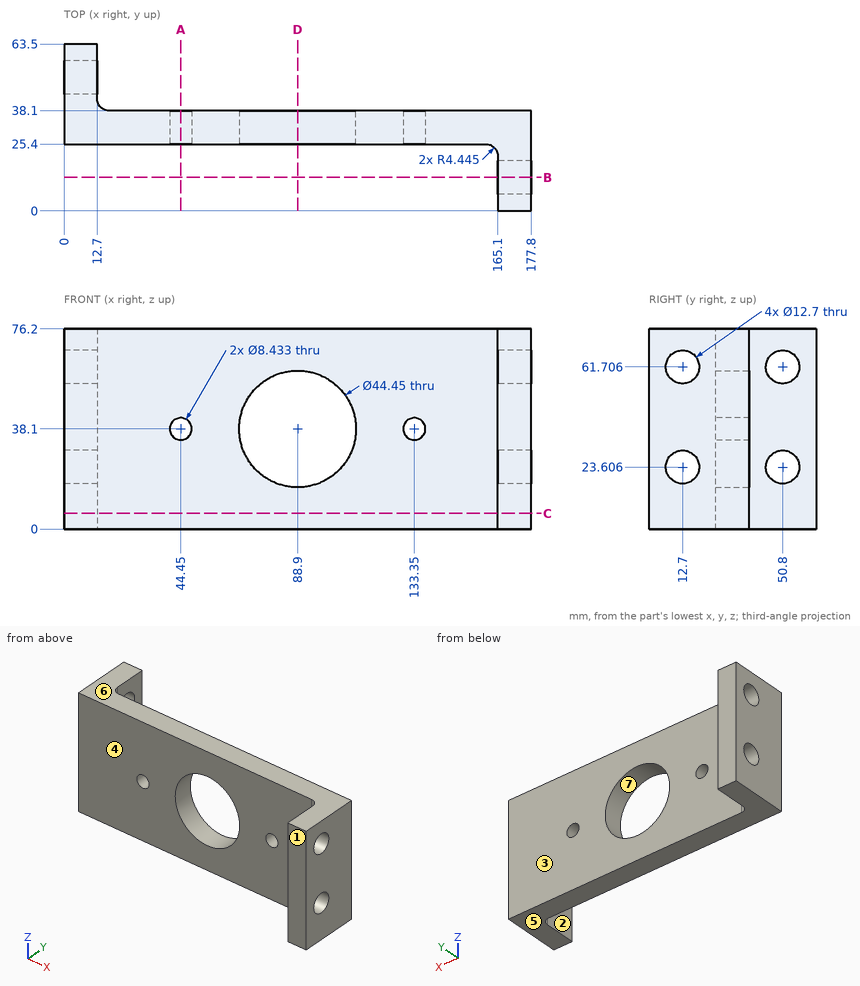
Part print with two shaded views. Sizes in mm from the minimum x, y, z corner. A direction names the side the tool comes from. Coordinates: 2 decimals unless noted, no trailing zeros. Write each loop counter-clockwise with the first axis right and the second up, starting at its lowest first coordinate (ties: lowest second). Pieces come first, ordered by that corner, then holes. Notation, with made-up numbers: (43, 21.25) - (75, 21.25) arc R23 ccw to (75, 32.25) - close; hole circle Ø4 at (42, 2). An arc over 180 degrees is marked (long way). Use a Markdown table: item, result. Add a question column.
Item 1: Band-saw the part on D-D, the plane x = 88.9. Write the cut outline in (y, z) (1 decimal).
Item 2: Band-saw the part on B-B, the plane y = 12.7. Write the cut outline in (x, z).
Item 3: Drill centre lines: line 1 along Z through (x, y) = (173, 12) (1 decimal); line 2 along X through (y, z) = (44.5, 48); line 3 along Y through (x, z) = (137, 19.5). Where is each one in solid material? Low to high.
Item 4: Band-saw the part on C-C, the plane z = 6. Write the cut outline in (x, y) (1 decimal), and give its area (3 significant figures).
Item 5: Band-saw the part on A-A, the plane x = 44.45. Write the cut outline in (y, z).
Item 6: 3-axis set-ups, long thin cutter, end or side, ignore diameter. For the marked faces 1, 2 and 3: which of +Z, -Z, +X, -X, +Y, -Y reach the whole face in a straight line?
Item 7: Drop flat-ended pins along their axis: pin 1 (16.5 mm diameter, centred on y = 12.7, z = 23.61, fed in from -X); pin 2 (1.5 mm diameter, centred on x = 123, z = 48.5, fed in from -Y); pin 3 (1.5 mm diameter, centred on x = 152.5, z = 66.5, fed in from +Y). Give the stop position or say it passes through.
Item 8: Two-plate mould, pull along Z, no slides. Class the marked faces 4, 5, 6 and 7: pulls with the +Z half, pulls with the -Z half, needs draft (parallel to the pull), parting line crosses it, or undercut.
A:
| question | item | result |
|---|---|---|
| 1 | outline | (25.4, 0) - (38.1, 0) - (38.1, 15.9) - (25.4, 15.9) - close; (25.4, 60.3) - (38.1, 60.3) - (38.1, 76.2) - (25.4, 76.2) - close |
| 2 | outline | (165.1, 0) - (177.8, 0) - (177.8, 17.26) - (165.1, 17.26) - close; (165.1, 29.96) - (177.8, 29.96) - (177.8, 55.36) - (165.1, 55.36) - close; (165.1, 68.06) - (177.8, 68.06) - (177.8, 76.2) - (165.1, 76.2) - close |
| 3 | line 1 | z = 0 to 17.3, 29.9 to 55.4, 68 to 76.2 |
| 3 | line 2 | x = 0 to 12.7 |
| 3 | line 3 | y = 25.4 to 38.1 |
| 4 | outline | (0, 25.4) - (160.7, 25.4) arc R4.4 cw to (165.1, 21) - (165.1, 0) - (177.8, 0) - (177.8, 38.1) - (17.1, 38.1) arc R4.4 cw to (12.7, 42.5) - (12.7, 63.5) - (0, 63.5) - close |
| 4 | area | 2,910 mm² |
| 5 | outline | (25.4, 0) - (38.1, 0) - (38.1, 33.88) - (25.4, 33.88) - close; (25.4, 42.32) - (38.1, 42.32) - (38.1, 76.2) - (25.4, 76.2) - close |
| 6 | face 1 | +Z, -Z, +X, -X, -Y |
| 6 | face 2 | +Z, -Z, -X, -Y |
| 6 | face 3 | +Z, -Z, +X, +Y |
| 7 | pin 1 | stops at x = 165.1 |
| 7 | pin 2 | stops at y = 25.4 |
| 7 | pin 3 | stops at y = 38.1 |
| 8 | face 4 | needs draft |
| 8 | face 5 | pulls with the -Z half |
| 8 | face 6 | pulls with the +Z half |
| 8 | face 7 | undercut |
